Build history of the part. All positions in model axes, mm. A direction names the side the tool comes from. Give positions to 0.01 mm unless a question says otherwise; leave off trailing zeros. Loops run counter-clockwise (first coordinate to the right, second up) from the corner with the lowest first, then second, coordinate; pieces in that order, holes last.
1) 3-axis set-ups, long thin cutter, end or side, ignore diameter. For faces 4 (the flat face through (1, 2, 1)), 5 (the flat face through (0.25, 0, 6)), 6 (the flat face through (1, 0, 7)): which of +Z, -Z, +X, -X, +Y, -Y reach the whole face in a straight line?
2) Band-saw the part on B-B on z = 6. List the corners of the cut face in (x, y) (3 decimals).
3) Wall check: line 1 (Z direction, x = -1.75, y = 3.25); line 2 (X direction, y = -1, z = 6.25); line 3 (Y direction, x = 1.5, z = 0.5). Give the ranges that are in metal, low to high.
4) Band-saw the part on A-A on y = 0. List the corners of the cut face in (x, z) (3 decimals).
5) Band-saw the part on D-D on z = 1.5. List the corners of the cut face in (x, y) (3 decimals), then the cut area to 3 significant figures.
6) Flat gauge pins, fed straight in: P1, Ø1, axis at y = 0.5, z = 6.5, coming from the +X side (3 decimals); P2, Ø1, axis at x = 1, z = 4.5, coming from the +Y side; P3, Ø2, axis at y = 0, z = 6, coming from the -X side (3 decimals). Where does each tip first touch, or does it go through?
7) Band-saw the part on C-C on x = 0. List the corners of the cut face in (y, z) (3 decimals), then the cut area to 3 significant figures.
8) Two-plate mould, pull along X, no slides. Class faces 1 (the cylindrical face through (-0.41, -1.83, 3.96)), 2 (the flat face through (-0.25, 0, 6)), 3 (the flat face through (0, 0, 0)): +X half, -X half, draft (parallel to the pull), parting line (faces both ways), or undercut.
```python
from build123d import *

# Parameters (mm, degrees)
F0_R     = 1.875
F1_DEPTH = 7
F0_R_2   = 3.75
F2_DEPTH = 1
F4_DEPTH = 2


with BuildPart() as f1:
    # F0 (on Top) → F1 (new body)
    with BuildSketch(Plane.XY):
        Circle(F0_R)
    extrude(amount=F1_DEPTH)

    # F0 (on Top) → F2 (join)
    with BuildSketch(Plane.XY):
        Circle(F0_R_2)
        Circle(F0_R, mode=Mode.SUBTRACT)
    extrude(amount=F2_DEPTH)

    # F3 (on face) → F4 (cut)
    with BuildSketch(Plane.XY.offset(7)):
        with BuildLine():
            Line((-0.25, 1.8582585934), (-0.25, -1.8582585934))
            ThreePointArc((-0.25, -1.8582585934), (0, -1.875), (0.25, -1.8582585934))
            Line((0.25, -1.8582585934), (0.25, 1.8582585934))
            ThreePointArc((0.25, 1.8582585934), (0, 1.875), (-0.25, 1.8582585934))
        make_face()
        with BuildLine():
            Line((-0.25, 2.5), (-0.25, 1.8582585934))
            ThreePointArc((-0.25, 1.8582585934), (0, 1.875), (0.25, 1.8582585934))
            Line((0.25, 1.8582585934), (0.25, 2.5))
            Line((0.25, 2.5), (-0.25, 2.5))
        make_face()
    extrude(amount=-F4_DEPTH, mode=Mode.SUBTRACT)


solid = f1.part
```
Findings below:
1. face 4: +Z
1. face 5: +Z, +Y, -Y
1. face 6: +Z, +X, -X, +Y, -Y
2. outline: (-0.25, -1.858) - (-0.25, 1.858) arc R1.875 ccw to start; (0.25, -1.858) arc R1.875 ccw to (0.25, 1.858) - close
3. line 1: z = 0 to 1
3. line 2: x = -1.59 to -0.25, 0.25 to 1.59
3. line 3: y = -3.44 to 3.44
4. outline: (-3.75, 0) - (3.75, 0) - (3.75, 1) - (1.875, 1) - (1.875, 7) - (0.25, 7) - (0.25, 5) - (-0.25, 5) - (-0.25, 7) - (-1.875, 7) - (-1.875, 1) - (-3.75, 1) - close
5. outline: circle Ø3.75 at (0, 0)
5. area: 11.0 mm2
6. P1: stops at x = 1.875
6. P2: stops at y = 1.81
6. P3: stops at x = -1.875
7. outline: (-3.75, 0) - (3.75, 0) - (3.75, 1) - (1.875, 1) - (1.875, 5) - (-1.875, 5) - (-1.875, 1) - (-3.75, 1) - close
7. area: 22.5 mm2
8. face 1: parting line
8. face 2: undercut
8. face 3: draft
